Input: part model. Units: mm. Frame: model coordinates. Give positions to 0.01 mm unless a question says otherwise; leave off trailing zeros. Write each loop counter-clockwise with the first axis right and the second up, starting at its lowest first coordinate (ties: lowest second). Pieces come first, ordered by that corner, then holes.
```python
from build123d import *

# Parameters (mm, degrees)
SKETCH1_W            = 240
SKETCH1_H            = 245
BOSS_EXTRUDE1_DEPTH  = 1.2
M3_CLEARANCE_HOLE1_D = 3.4
M5_CLEARANCE_HOLE1_D = 5.5


with BuildPart() as part:
    # Sketch1 → Boss-Extrude1 (new body)
    with BuildSketch(Plane(origin=(0, 0, 0), x_dir=(1, 0, 0), z_dir=(0, 1, 0))):
        Rectangle(SKETCH1_W, SKETCH1_H)
    extrude(amount=BOSS_EXTRUDE1_DEPTH)

    # M3 Clearance Hole1 (through all)
    with Locations(Plane(origin=(0, 1.2, 0), x_dir=(1, 0, 0), z_dir=(0, 1, 0))):
        with Locations((0, 0), (105, 105), (-105, -105), (-105, 105), (105, -105)):
            Hole(M3_CLEARANCE_HOLE1_D / 2)

    # M5 Clearance Hole1 (through all)
    with Locations(Plane(origin=(0, 0, 0), x_dir=(-1, 0, 0), z_dir=(0, -1, 0))):
        with Locations((-112.5, -114), (112.5, 114), (112.5, -114), (-112.5, 114)):
            Hole(M5_CLEARANCE_HOLE1_D / 2)


solid = part.part
```
Item 1: Ray query, line 1 (X direction, y = 0.3, z = 114); line 2 (Z direction, x = -112.5, y = 0.5); line 3 (Z direction, x = -105, y = 0.9). Return the intervals inside material, ascending.
Item 2: Section A-A (x = -112.5). Return loops of the section in (y, z).
Item 3: Mould query, pull axis Z, two halves, no side actions, for faces 1 (the flat face through (-2, 1.2, -2)), 2 (the cylindrical face through (-113.096, 0.608, -111.315)). Classes: +Z half, -Z half, draft (parallel to the pull), parting line (faces both ways), or undercut.
Solved:
1. line 1: x = -120 to -115.25, -109.75 to 109.75, 115.25 to 120
1. line 2: z = -122.5 to -116.75, -111.25 to 111.25, 116.75 to 122.5
1. line 3: z = -122.5 to -106.7, -103.3 to 103.3, 106.7 to 122.5
2. outline: (0, -122.5) - (1.2, -122.5) - (1.2, -116.75) - (0, -116.75) - close; (0, -111.25) - (1.2, -111.25) - (1.2, 111.25) - (0, 111.25) - close; (0, 116.75) - (1.2, 116.75) - (1.2, 122.5) - (0, 122.5) - close
3. face 1: draft
3. face 2: undercut
